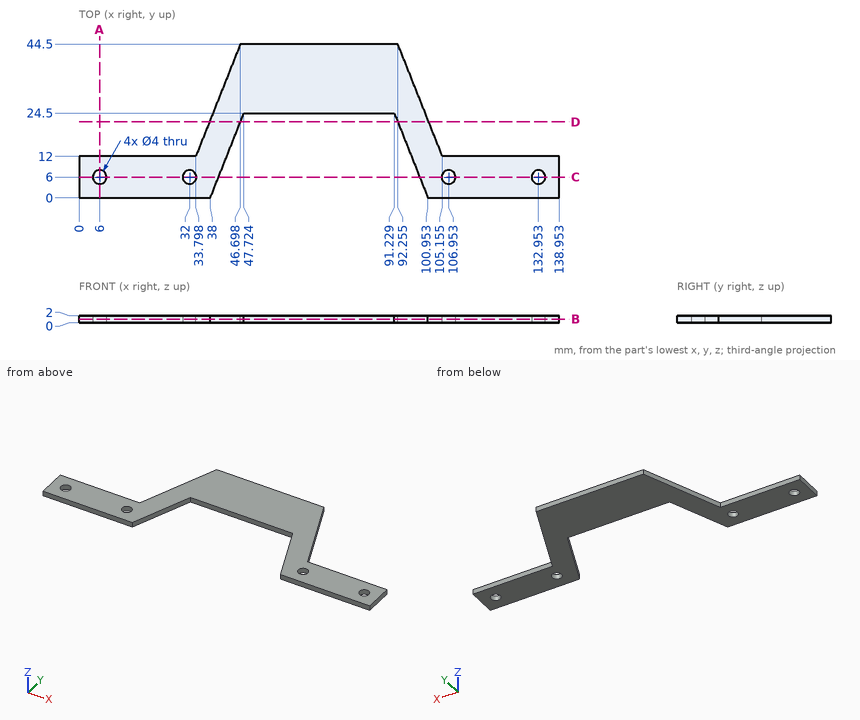
Design review of the part shown in the three views and the two pictorial views. Dimensions are in mm from the part's minimum x, y and z. Give positions to 0.01 mm unless a question says otherwise; leave off trailing zeros. Write each loop counter-clockwise with the first axis right and the second up, starting at its lowest first coordinate (ties: lowest second). Pieces come first, ordered by that corner, then holes. Notation, with made-up numbers: (-33, -34) -> (6, -34) arc R23 cw to (6, -26) -> close; hole circle Ø1 at (30, 36.5). An arc over 180 degrees is marked (long way). Answer in a Markdown table with one row per item.
1) Add section C-C on y = 6. State the section outline as (x, z) points.
Worked answers:
| item | result |
|---|---|
| outline | (0, 0) -> (4, 0) -> (4, 2) -> (0, 2) -> close; (8, 0) -> (30, 0) -> (30, 2) -> (8, 2) -> close; (34, 0) -> (40.38, 0) -> (40.38, 2) -> (34, 2) -> close; (98.57, 0) -> (104.95, 0) -> (104.95, 2) -> (98.57, 2) -> close; (108.95, 0) -> (130.95, 0) -> (130.95, 2) -> (108.95, 2) -> close; (134.95, 0) -> (138.95, 0) -> (138.95, 2) -> (134.95, 2) -> close |
2) Clearance check with a flat-ended pin moving along its axis: P1, Ø0.6, axis at x = 17, z = 0.5, coming from the +Y side. State where the tip first meets the part, or that it passes through.
Worked answers:
| item | result |
|---|---|
| P1 | y = 12 |
3) Add section B-B on z = 1.05. State the section outline as (x, y) points (1 decimal).
Worked answers:
| item | result |
|---|---|
| outline | (0, 0) -> (38, 0) -> (47.7, 24.5) -> (91.2, 24.5) -> (101, 0) -> (139, 0) -> (139, 12) -> (105.2, 12) -> (92.3, 44.5) -> (46.7, 44.5) -> (33.8, 12) -> (0, 12) -> close; hole circle Ø4 at (6, 6); hole circle Ø4 at (32, 6); hole circle Ø4 at (107, 6); hole circle Ø4 at (133, 6) |
4) Add section A-A on x = 6. State the section outline as (y, z) points.
Worked answers:
| item | result |
|---|---|
| outline | (0, 0) -> (4, 0) -> (4, 2) -> (0, 2) -> close; (8, 0) -> (12, 0) -> (12, 2) -> (8, 2) -> close |
5) Add section D-D on y = 22. State the section outline as (x, z) points (1 decimal).
Worked answers:
| item | result |
|---|---|
| outline | (37.8, 0) -> (46.7, 0) -> (46.7, 2) -> (37.8, 2) -> close; (92.2, 0) -> (101.2, 0) -> (101.2, 2) -> (92.2, 2) -> close |
6) For L1, parallel to Y at x = 6, z = 1.4; L2, parallel to Y at x = 112.5, z = 0.65; L3, parallel to Y at x = 108, z = 1.05 (1 decimal), list the stretches that pass through material, from the lowest coordinate up. Write a range as [from, to].
Worked answers:
| item | result |
|---|---|
| L1 | [0, 4], [8, 12] |
| L2 | [0, 12] |
| L3 | [0, 4.3], [7.7, 12] |
